Autodesk Inventor part; units mm, degrees
ref_plane "Work Plane1" through (0, 0, 141.7574) normal (0, 0, 1) x (1, 0, 0)
ref_plane "Work Plane2" through (0, 0, 103.6574) normal (0, 0, 1) x (1, 0, 0)
ref_plane "Work Plane3" through (0, 0, 0) normal (0, 0, -1) x (-1, 0, 0)
sketch "Sketch1" plane through (0, 0, 0) normal (0, 0, 1) x (1, 0, 0)
  circle A0 centre (0, 0) radius 7.8994
  circle A1 centre (0, 0) radius 10.668
  dimension "d0" = 15.7988
  dimension "d1" = 21.336
extrude "Extrusion1" add sketch "Sketch1" along normal blind 141.7574
ref_plane "Work Plane1" through (0, 0, 141.7574) normal (0, 0, 1) x (1, 0, 0)
ref_plane "Work Plane2" through (0, 0, 103.6574) normal (0, 0, 1) x (1, 0, 0)
sketch "Sketch2" plane through (0, 0, 103.6574) normal (0, 0, 1) x (1, 0, 0)
  line L0 (-1.32, 11.5038) -> (1.3938, 11.5038)
  line L1 (1.3938, 11.5038) -> (1.3938, -14.9502)
  line L2 (1.3938, -14.9502) -> (-1.32, -14.9502)
  line L3 (-1.32, -14.9502) -> (-1.32, 11.5038)
  point P0 (0, 0)
extrude "Extrusion2" cut sketch "Sketch2" along normal mid plane 3.175
ref_plane "Work Plane3" through (0, 0, 0) normal (0, 0, -1) x (-1, 0, 0)
ref_plane "Work Plane4" through (0, 0, 69.85) normal (0, 0, -1) x (-1, 0, 0)
mirror "Mirror1" about plane through (0, 0, 69.85) normal (0, 0, -1) of "Extrusion2"
properties part number "custom pvc spool"
Can you work these out from the model? Positions are in its coordinate system, mm. A direction names the side the tool comes from. Round coordinates to 2 decimals unless told otherwise and drop trailing zeros. Order: outer loops, then holes, each group sorted by start corner. A loop starts at its lowest first (then second) coordinate and runs counter-clockwise, first axis right, second up. Notation, with made-up numbers: (-13, 4) - (-4, 4) arc R16 cw to (-4, 10) - close; hole circle Ø10 at (-35, -11.5). An arc over 180 degrees is marked (long way). Answer in a Markdown table with one row per item.
(1) For P1, Ø3, axis at y = 5.5, z = 66, coming from the +X side; P2, Ø10, axis at x = -7.5, z = 113.5, coming from the -Y side; P3, Ø8, axis at x = 5, z = 111.5, coming from the +Y side; P4, Ø1.4, axis at x = -0.5, y = 10, coming from the -Z side, each with a flat end and sliding along its axis, tell me the tip position at first contact or that it passes through.
From the geometry:
| item | result |
|---|---|
| P1 | stops at x = 9.89 |
| P2 | stops at y = -10.37 |
| P3 | stops at y = 10.62 |
| P4 | stops at z = 0 |
(2) Suppose I cut it at C-C, the plane z = 69. Please give me the cut outline in (x, y), plus the area to 3 significant figures.
From the geometry:
| item | result |
|---|---|
| outline | circle Ø21.34 at (0, 0); hole circle Ø15.8 at (0, 0) |
| area | 161 mm2 |
(3) Please list where these lines run through material, in increasing order: L1, parallel to Y at x = 0, z = 95.5; L2, parallel to Y at x = 1.5, z = 30.5; L3, parallel to X at y = 2.5, z = 132. Write a range as from..to.
From the geometry:
| item | result |
|---|---|
| L1 | y = -10.67..-7.9, 7.9..10.67 |
| L2 | y = -10.56..-7.76, 7.76..10.56 |
| L3 | x = -10.37..-7.49, 7.49..10.37 |
(4) Suppose I cut it at B-B, the plane y = 0. Please give me the cut outline in (x, z), plus the area to 3 significant figures.
From the geometry:
| item | result |
|---|---|
| outline | (-10.67, 0) - (-7.9, 0) - (-7.9, 141.76) - (-10.67, 141.76) - close; (7.9, 0) - (10.67, 0) - (10.67, 141.76) - (7.9, 141.76) - close |
| area | 785 mm2 |
(5) Suppose I cut it at A-A, the plane x = 0. Please give me the cut outline in (y, z).
From the geometry:
| item | result |
|---|---|
| outline | (-10.67, 0) - (-7.9, 0) - (-7.9, 34.46) - (-10.67, 34.46) - close; (-10.67, 37.63) - (-7.9, 37.63) - (-7.9, 102.07) - (-10.67, 102.07) - close; (-10.67, 105.24) - (-7.9, 105.24) - (-7.9, 141.76) - (-10.67, 141.76) - close; (7.9, 0) - (10.67, 0) - (10.67, 34.46) - (7.9, 34.46) - close; (7.9, 37.63) - (10.67, 37.63) - (10.67, 102.07) - (7.9, 102.07) - close; (7.9, 105.24) - (10.67, 105.24) - (10.67, 141.76) - (7.9, 141.76) - close |
(6) Which directions (+Z, -Z, +X, -X, +Y, -Y) give clear straight access to the entire face, cutting with the end or side of a thin tool? Please do faces 1 (the face through (-7.89, -0.35, 69.89)), 2 (the face through (0, -9, 34.455)).
From the geometry:
| item | result |
|---|---|
| face 1 | +Z, -Z |
| face 2 | +Y, -Y |
(7) If we mould it in two halves opening along X, with no side actions, what happens to faces 3 (the face through (-1.32, 9, 104)), 4 (the face through (-7, -4, 141.757)), 5 (the face through (4.923, 9.464, 69.886))? For each: released by +X, released by -X, zero draft, split by the parting line, or undercut.
From the geometry:
| item | result |
|---|---|
| face 3 | undercut |
| face 4 | zero draft |
| face 5 | split by the parting line |
